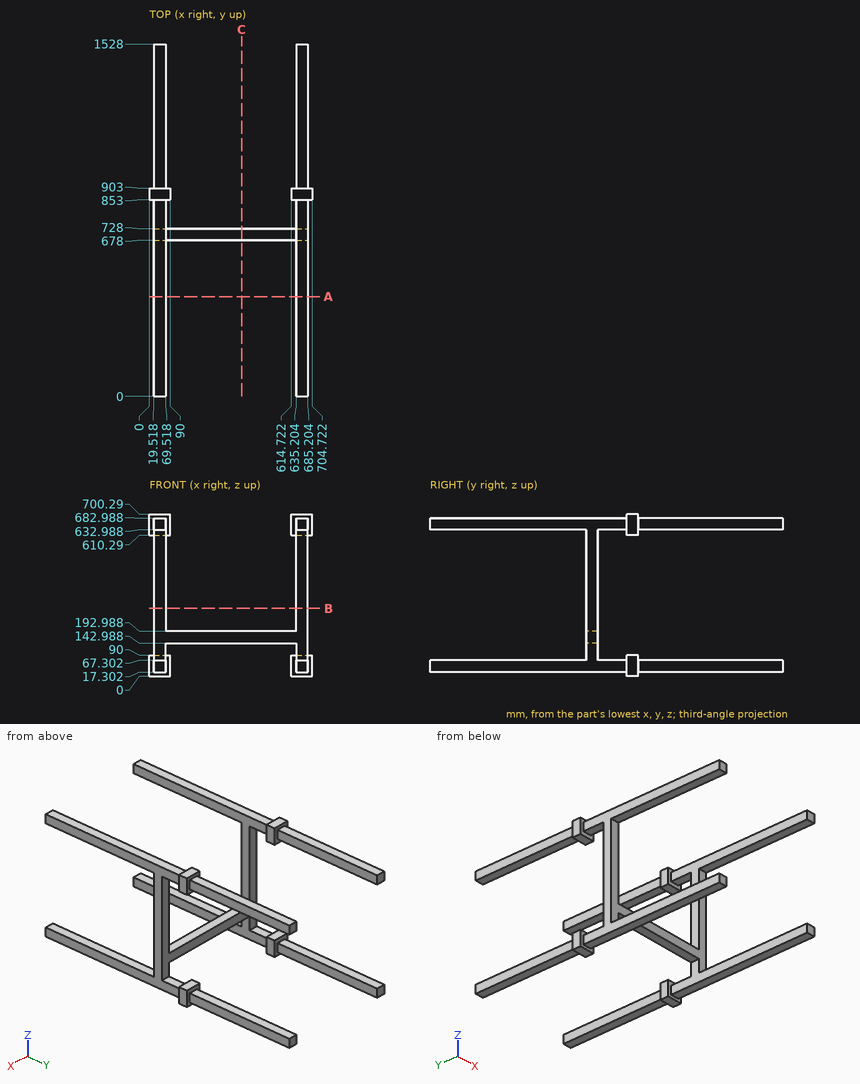
Design review of the part shown in the three views and the two pictorial views. Dimensions are in mm from the part's minimum x, y and z. Round coordinates to 2 decimals unless told otherwise and drop trailing zeros. Loops run counter-clockwise (first coordinate to the right, second up) from the corner with the lowest first, then second, coordinate; pieces in that order, holes last. Notation, with made-up numbers: (31, -16.5) -> (37, -16.5) arc R26 ccw to (37, -2.5) -> close; hole circle Ø7 at (-8, -14.5). An arc over 180 degrees is marked (long way). Answer as CSV lines item,"result".
1) Add section B-B on z = 293. Write out the cut boundary in (x, y), plus the area to 3 significant figures.
Geometry results:
outline,"(19.52, 678) -> (69.52, 678) -> (69.52, 728) -> (19.52, 728) -> close; (635.2, 678) -> (685.2, 678) -> (685.2, 728) -> (635.2, 728) -> close"
area,"5,000 mm²"
2) Add section A-A on y = 433. Write out the cut boundary in (x, z).
Geometry results:
outline,"(19.52, 17.3) -> (69.52, 17.3) -> (69.52, 67.3) -> (19.52, 67.3) -> close; (19.52, 632.99) -> (69.52, 632.99) -> (69.52, 682.99) -> (19.52, 682.99) -> close; (635.2, 17.3) -> (685.2, 17.3) -> (685.2, 67.3) -> (635.2, 67.3) -> close; (635.2, 632.99) -> (685.2, 632.99) -> (685.2, 682.99) -> (635.2, 682.99) -> close"
3) For P1, Ø25, axis at x = 653.5, y = 279, coming from the +Z side; P2, Ø4, axis at x = 304.5, z = 180, coming from the +Y side, all flat-tipped, find the tip position at first contact; note any pin that passes through.
Geometry results:
P1,"stops at z = 682.99"
P2,"stops at y = 728"
4) To check wall thickness, follow line 1 along X through (y, z) = (853.5, 35.5); line 2 along X through (y, z) = (524.5, 53.5); line 3 along Z through (x, y) = (350, 721.5). State the ranges of each line that lie inside material, in increasing order. Write a range as from..to.
Geometry results:
line 1,"x = 0..90, 614.72..704.72"
line 2,"x = 19.52..69.52, 635.2..685.2"
line 3,"z = 142.99..192.99"
5) Add section C-C on x = 399. Write out the cut boundary in (y, z).
Geometry results:
outline,"(678, 142.99) -> (728, 142.99) -> (728, 192.99) -> (678, 192.99) -> close"
